Geometry check sheet. Reference: the model listing, model coordinates, mm. Face numbers are marked on the shaded views. A direction names the side the tool comes from. Round coordinates to 2 decimals unless told otherwise and drop trailing zeros. Order: outer loops, then holes, each group sorted by start corner. A loop starts at its lowest first (then second) coordinate and runs counter-clockwise, first axis right, second up. Notation, with made-up numbers: (79, -2.5) -> (108, -2.5) arc R17 ccw to (108, 3.5) -> close; hole circle Ø4 at (53, 26). An arc over 180 degrees is marked (long way). Use a Markdown table: item, result. Add a question column.
Item 1: Sectioned sample at D-D, the plane z = 5. Record the cut outline in (x, y), and give its area (3 significant figures).
Item 2: Set-up check for the marked faces 1 and 2: record each of +Z, -Z, +X, -X, +Y, -Y from which the full face is reachable in a straight line by a thin tool's end or side.
Item 3: Material ranges on probe 1 along Z at (x, y) = (27, 0); probe 2 along X at (y, z) = (3.5, 16.5); probe 3 along X at (y, z) = (-2.5, -6.5), recorded low to high. Write a range as [from, to].
Item 4: Sectioned sample at A-A, the plane y = 0. Record the cut outline in (x, z), and give its area (3 significant figures).
Item 5: Sectioned sample at C-C, the plane x = 65. Record the cut outline in (y, z).
Item 6: Gauge pin test, flat ends, axial feed: pin 1 Ø2.5 at (y, z) = (0, 13.5) entering from -X; pin 2 Ø4 at (x, y) = (100.5, -4.5) entering from +Z; pin 3 Ø5 at (y, z) = (2.5, 11.5) entering from -X; pin 4 Ø17.5 at (y, z) = (2.5, -0.5) entering from -X. Record the tip position at first contact, or that the pin passes through.
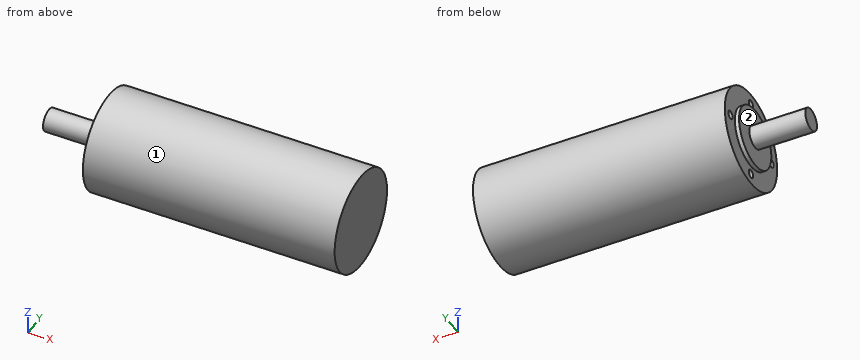
from build123d import *

# Parameters (mm, degrees)
SKETCH2_R          = 1.5
CUT_EXTRUDE1_DEPTH = 10


with BuildPart() as part:
    # Sketch1 → Revolve1 (revolve)
    with BuildSketch(Plane.XY):
        Polygon((0, 0), (0, 4), (20, 4), (20, 11), (21.5, 11), (21.5, 17.85), (111.5, 17.85), (111.5, 0), align=None)
    revolve(axis=Axis((111.5, 0, 0), (-1, 0, 0)))

    # Sketch2 → Cut-Extrude1 (cut)
    with BuildSketch(Plane.ZY.offset(-21.5)):
        with Locations(Location((0, 14, 0), (0, 0, 270))):
            Circle(SKETCH2_R)
        with Locations(Location((14, 0, 0), (0, 0, 270))):
            Circle(SKETCH2_R)
        with Locations(Location((0, -14, 0), (0, 0, 270))):
            Circle(SKETCH2_R)
        with Locations(Location((-14, 0, 0), (0, 0, 270))):
            Circle(SKETCH2_R)
    extrude(amount=-CUT_EXTRUDE1_DEPTH, mode=Mode.SUBTRACT)


solid = part.part
Found:
| question | item | result |
|---|---|---|
| 1 | outline | (20, -9.8) -> (21.5, -9.8) -> (21.5, -17.14) -> (111.5, -17.14) -> (111.5, 17.14) -> (21.5, 17.14) -> (21.5, 9.8) -> (20, 9.8) -> close |
| 1 | area | 3,110 mm2 |
| 2 | face 1 | +X, -X |
| 2 | face 2 | -X |
| 3 | probe 1 | z = [-17.85, -15.5], [-12.5, 12.5], [15.5, 17.85] |
| 3 | probe 2 | x = [21.5, 111.5] |
| 3 | probe 3 | x = [20, 111.5] |
| 4 | outline | (0, -4) -> (20, -4) -> (20, -11) -> (21.5, -11) -> (21.5, -12.5) -> (31.5, -12.5) -> (31.5, -15.5) -> (21.5, -15.5) -> (21.5, -17.85) -> (111.5, -17.85) -> (111.5, 17.85) -> (21.5, 17.85) -> (21.5, 15.5) -> (31.5, 15.5) -> (31.5, 12.5) -> (21.5, 12.5) -> (21.5, 11) -> (20, 11) -> (20, 4) -> (0, 4) -> close |
| 4 | area | 3,350 mm2 |
| 5 | outline | circle Ø35.7 at (0, 0) |
| 6 | pin 1 | stops at x = 21.5 |
| 6 | pin 2 | stops at z = 17.67 |
| 6 | pin 3 | stops at x = 20 |
| 6 | pin 4 | stops at x = 0 |
